The model under review builds one solid part; all positions refer to its coordinate system, in mm. Coordinates: 2 decimals unless noted, no trailing zeros. Order: outer loops, then holes, each group sorted by start corner. A loop starts at its lowest first (then second) coordinate and runs counter-clockwise, first axis right, second up. Notation, with made-up numbers: (62, 44.25) - (68, 44.25) arc R31 cw to (68, 69.25) - close; hole circle Ø10 at (49.25, -17.75). An arc over 180 degrees is marked (long way). Answer in a Markdown table with one row per item.
```python
from build123d import *

# Parameters (mm, degrees)
SKETCH1_W           = 368
SKETCH1_H           = 278
BOSS_EXTRUDE1_DEPTH = 39
SKETCH2_W           = 368
SKETCH2_H           = 278
SKETCH2_W_2         = 325
SKETCH2_H_2         = 250
CUT_EXTRUDE1_DEPTH  = 21
SKETCH3_W           = 325
SKETCH3_H           = 250
SKETCH3_W_2         = 247
SKETCH3_H_2         = 200
CUT_EXTRUDE2_DEPTH  = 7
SKETCH4_R           = 3
CUT_EXTRUDE3_DEPTH  = 59


with BuildPart() as part:
    # Sketch1 → Boss-Extrude1 (new body)
    with BuildSketch(Plane(origin=(0, 0, 0), x_dir=(1, 0, 0), z_dir=(0, 1, 0))):
        with Locations((184, 139)):
            Rectangle(SKETCH1_W, SKETCH1_H)
    extrude(amount=-BOSS_EXTRUDE1_DEPTH)

    # Sketch2 → Cut-Extrude1 (cut)
    with BuildSketch(Plane(origin=(0, 0, 0), x_dir=(1, 0, 0), z_dir=(0, 1, 0))):
        with Locations((184, 139)):
            Rectangle(SKETCH2_W, SKETCH2_H)
        with Locations((184, 139)):
            Rectangle(SKETCH2_W_2, SKETCH2_H_2, mode=Mode.SUBTRACT)
    extrude(amount=-CUT_EXTRUDE1_DEPTH, mode=Mode.SUBTRACT)

    # Sketch3 → Cut-Extrude2 (cut)
    with BuildSketch(Plane(origin=(0, 0, 0), x_dir=(1, 0, 0), z_dir=(0, 1, 0))):
        with Locations((184, 139)):
            Rectangle(SKETCH3_W, SKETCH3_H)
        with Locations((184, 139)):
            Rectangle(SKETCH3_W_2, SKETCH3_H_2, mode=Mode.SUBTRACT)
    extrude(amount=-CUT_EXTRUDE2_DEPTH, mode=Mode.SUBTRACT)

    # Sketch4 → Cut-Extrude3 (cut)
    with BuildSketch(Plane(origin=(0, 0, 0), x_dir=(1, 0, 0), z_dir=(0, 1, 0))):
        with Locations(Location((9, 150.3, 0), (0, 0, 270))):
            Circle(SKETCH4_R)
        with Locations(Location((359, 150.3, 0), (0, 0, 270))):
            Circle(SKETCH4_R)
    extrude(amount=-CUT_EXTRUDE3_DEPTH, mode=Mode.SUBTRACT)


solid = part.part
```
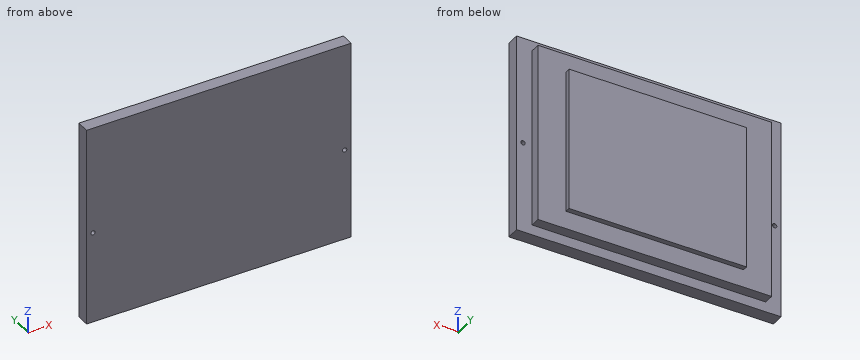
Item 1: We need section D-D, the plane x = 300. Write out the cut boundary in (y, z).
Check values:
| item | result |
|---|---|
| outline | (-39, -278) - (-21, -278) - (-21, -264) - (-7, -264) - (-7, -239) - (0, -239) - (0, -39) - (-7, -39) - (-7, -14) - (-21, -14) - (-21, 0) - (-39, 0) - close |
Item 2: We need section C-C, the plane z = -30. Write out the cut boundary in (x, y), then the cut area to 3 significant figures.
Check values:
| item | result |
|---|---|
| outline | (0, -39) - (368, -39) - (368, -21) - (346.5, -21) - (346.5, -7) - (21.5, -7) - (21.5, -21) - (0, -21) - close |
| area | 11,200 mm^2 |
Item 3: To check wall thickness, follow line 1 (X direction, y = -29, z = -150); line 2 (Z direction, x = 359, y = -30.75); line 3 (Z direction, x = 68, y = -2.5). State the ranges of each line that lie inside material, in increasing order. Write a range as from..to.
Check values:
| item | result |
|---|---|
| line 1 | 0..6.02, 11.98..356.02, 361.98..368 |
| line 2 | -278..-153.3, -147.3..0 |
| line 3 | -239..-39 |
Item 4: We need section B-B, the plane z = -63.5. Write out the cut boundary in (x, y).
Check values:
| item | result |
|---|---|
| outline | (0, -39) - (368, -39) - (368, -21) - (346.5, -21) - (346.5, -7) - (307.5, -7) - (307.5, 0) - (60.5, 0) - (60.5, -7) - (21.5, -7) - (21.5, -21) - (0, -21) - close |
Item 5: We need section A-A, the plane x = 43. Write out the cut boundary in (y, z), then the cut area to 3 significant figures.
Check values:
| item | result |
|---|---|
| outline | (-39, -278) - (-21, -278) - (-21, -264) - (-7, -264) - (-7, -14) - (-21, -14) - (-21, 0) - (-39, 0) - close |
| area | 8,500 mm^2 |
Item 6: Clearance check with flat-ended pins moving along their axes: pin 1 Ø5 at (x, y) = (121.5, -30.5) entering from +Z; pin 2 Ø5.5 at (y, z) = (-3.5, -92) entering from +X; pin 3 Ø7.5 at (y, z) = (-4.5, -107) entering from -X; pin 4 Ø3.5 at (x, y) = (208, -2) entering from -Z. State where each tip first meets the part, or that it passes through.
Check values:
| item | result |
|---|---|
| pin 1 | z = 0 |
| pin 2 | x = 307.5 |
| pin 3 | x = 21.5 |
| pin 4 | z = -239 |
